Source: CAD feature listing. Evaluate the final solid. Frame: model axes, mm. A direction names the side the tool comes from. Round coordinates to 2 decimals unless told otherwise and drop trailing zeros. Write each loop counter-clockwise with the first axis right and the second up, starting at its lowest first coordinate (ties: lowest second). Pieces come first, ordered by that corner, then holes.
```python
from build123d import *

# Parameters (mm, degrees)
F0_R      = 27.305
F0_R_2    = 7.14375
F1_DEPTH  = 4.699
F2_R      = 17.018
F2_R_2    = 7.14375
F3_DEPTH  = 2.921
F4_R      = 12.319
F4_R_2    = 7.14375
F5_DEPTH  = 4.4704
F6_SIZE2  = 1.524
F6_SIZE   = 1.524
F7_R      = 22.987
F7_R_2    = 11.938
F8_DEPTH  = 2.286
F10_D     = 1.778
F10_DEPTH = 5.9327142857
F10_TIP   = 0.5341650903
F11_D     = 3.5687
F12_D     = 2.9464


with BuildPart() as f1:
    # F0 (on Top) → F1 (new body)
    with BuildSketch(Plane.XY):
        Circle(F0_R)
        Circle(F0_R_2, mode=Mode.SUBTRACT)
    extrude(amount=F1_DEPTH)

    # F2 (on face) → F3 (join)
    with BuildSketch(Plane.XY.offset(4.699)):
        Circle(F2_R)
        Circle(F2_R_2, mode=Mode.SUBTRACT)
    extrude(amount=F3_DEPTH)

    # F4 (on face) → F5 (join)
    with BuildSketch(Plane.XY.offset(7.62)):
        Circle(F4_R)
        Circle(F4_R_2, mode=Mode.SUBTRACT)
    extrude(amount=F5_DEPTH)

    # F6
    f6_edges = [f1.edges().sort_by_distance(p)[0] for p in [
        (-12.319, 0, 12.0904),
    ]]
    chamfer(f6_edges, length=F6_SIZE, length2=F6_SIZE2)

    # F7 (on face) → F8 (cut)
    with BuildSketch(Plane(origin=(0, 0, 0), x_dir=(1, 0, 0), z_dir=(0, 0, -1))):
        Circle(F7_R)
        Circle(F7_R_2, mode=Mode.SUBTRACT)
    extrude(amount=-F8_DEPTH, mode=Mode.SUBTRACT)

    # F10
    with Locations(Plane(origin=(0, 0, 0), x_dir=(1, 0, 0), z_dir=(0, 0, -1))):
        with Locations((-8.1389067448, 4.699), (-8.1334533724, -4.689554482), (8.1389067448, 4.699), (0, 0), (0.0054533724, 9.388554482), (0, -9.398), (8.128, -4.699)):
            Hole(F10_D / 2, depth=F10_DEPTH)
            with Locations((0, 0, -(F10_DEPTH + F10_TIP / 2))):  # 118° drill point
                Cone(0, F10_D / 2, F10_TIP, mode=Mode.SUBTRACT)

    # F11 (through all)
    with Locations(Plane(origin=(0, 0, 0), x_dir=(1, 0, 0), z_dir=(0, 0, -1))):
        with Locations((14.3764, 14.3764), (14.3764, -14.3764), (-14.3764, -14.3764), (-14.3764, 14.3764)):
            Hole(F11_D / 2)

    # F12 (through all)
    with Locations(Plane(origin=(0, 0, 0), x_dir=(1, 0, 0), z_dir=(0, 0, -1))):
        with Locations((12.573, 21.7678), (21.7678, 12.573), (21.7678, -12.573), (12.573, -21.7678), (-12.573, -21.7678), (-21.7678, -12.573), (-21.7678, 12.573), (-12.573, 21.7678)):
            Hole(F12_D / 2)


solid = f1.part
```
Q1. Section query C-C, the plane z = 8.75. Output: boundary loops of the cut face in (x, y).
Q2. Section query A-A, the plane y = 0. Output: boundary loops of the cut face in (x, z) (3 decimals), and give its area (3 significant figures).
Q3. Set-up query: faces 4 (the face through (9, 9, 7.62)), 5 (the face through (0, -8, 0)), 6 (the face through (-0.405, -8.6, 3.008)). Return all of +Z, -Z, +X, -X, +Y, -Y with unobstructed straight access to the full face (end or side cutting, diameter ignored); none if empty.
Q4. Section query B-B, the plane y = 15.5. Output: boundary loops of the cut face in (x, z).
Q5. Mould query, pull axis X, two halves, no side actions, for faces 1 (the face through (7, -2.2, 12.09)), 2 (the face through (-2.215, 16.873, 6.139)), 3 (the face through (7.307, 5.039, 3.008)). Classes: pulls with the +X half, pulls with the -X half, needs draft (parallel to the pull), parting line crosses it, or undercut.
Q6. Line query: line 1 (X direction, y = 22, z = 4.5); line 2 (Y direction, x = 8.5, z = 4); line 3 (Z direction, x = 10.5, y = 20.5). Output: solid intervals per line, ascending.
Q7. Pin query (flat end, axial travel): P1, Ø3, axis at x = 14.38, y = 14.38, coming from the +Z side; P2, Ø1, axis at x = 0.5, z = 7.5, coming from the +Y side; P3, Ø3, axis at x = -11, y = 2, coming from the -Z side; P4, Ø1.5, axis at y = -1.5, z = 8, coming from the -X side. Return the tip coordinate at first contact, or that it passes through.
Filled in:
1. outline: circle Ø24.64 at (0, 0); hole circle Ø14.29 at (0, 0)
2. outline: (-27.305, 0) - (-22.987, 0) - (-22.987, 2.286) - (-11.938, 2.286) - (-11.938, 0) - (-7.144, 0) - (-7.144, 12.09) - (-10.795, 12.09) - (-12.319, 10.566) - (-12.319, 7.62) - (-17.018, 7.62) - (-17.018, 4.699) - (-27.305, 4.699) - close; (7.144, 0) - (11.938, 0) - (11.938, 2.286) - (22.987, 2.286) - (22.987, 0) - (27.305, 0) - (27.305, 4.699) - (17.018, 4.699) - (17.018, 7.62) - (12.319, 7.62) - (12.319, 10.566) - (10.795, 12.09) - (7.144, 12.09) - close
2. area: 241 mm2
3. face 4: +Z
3. face 5: -Z, +X, -X, +Y, -Y
3. face 6: -Z
4. outline: (-22.48, 0) - (-16.98, 0) - (-16.98, 2.29) - (-15.76, 2.29) - (-15.76, 4.7) - (-22.48, 4.7) - close; (-12.99, 2.29) - (12.99, 2.29) - (12.99, 4.7) - (7.03, 4.7) - (7.03, 7.62) - (-7.03, 7.62) - (-7.03, 4.7) - (-12.99, 4.7) - close; (15.76, 2.29) - (16.98, 2.29) - (16.98, 0) - (22.48, 0) - (22.48, 4.7) - (15.76, 4.7) - close
5. face 1: needs draft
5. face 2: parting line crosses it
5. face 3: undercut
6. line 1: x = -16.17 to -14.03, -11.12 to 11.12, 14.03 to 16.17
6. line 2: y = -25.95 to -5.51, -3.89 to 3.89, 5.51 to 25.95
6. line 3: z = 0 to 4.7
7. P1: passes through
7. P2: stops at y = 17.02
7. P3: stops at z = 0
7. P4: stops at x = -17
